Autodesk Inventor part; units mm, degrees
ref_plane "XZ Plane" through (0, 0, 0) normal (0, 1, 0) x (-1, 0, 0)
ref_plane "XY Plane" through (0, 0, 0) normal (0, 0, 1) x (1, 0, 0)
sketch "Sketch1" plane through (0, 0, 0) normal (0, 0, 1) x (1, 0, 0)
  circle A0 centre (0, 0) radius 7.9375
  dimension "d0" = 15.875
extrude "Extrusion1" add sketch "Sketch1" along normal blind 58.039
sketch "Sketch2" plane through (0, 0, 0) normal (0, 0, -1) x (-1, 0, 0)
  circle A0 centre (0, 0) radius 82.55
  dimension "d3" = 165.1
extrude "Extrusion2" add sketch "Sketch2" along normal blind 45.4533
sketch "Sketch3" plane through (0, 0, -45.4533) normal (0, 0, -1) x (-1, 0, 0)
  circle A0 centre (0, 0) radius 67.2719
  circle A1 centre (0, 0) radius 53.975
  dimension "d6" = 134.5438
  dimension "d20" = 107.95
ref_plane "Work Plane3" through (0, 0, -45.4533) normal (0, 0, -1) x (-1, 0, 0)
sketch "Sketch4" plane through (0, 0, -45.4533) normal (0, 0, -1) x (-1, 0, 0)
  point P0 (0, 0)
ref_plane "Work Plane1" through (7.9375, 0, 0) normal (1, 0, 0) x (0, 1, 0)
sketch "Sketch5" plane through (7.9375, 0, 0) normal (1, 0, 0) x (0, 1, 0)
  line L0 (-7.9375, 0) -> (-7.9375, 58.039)
  line L1 (7.9375, 58.039) -> (-7.9375, 58.039)
  line L2 (7.9375, 58.039) -> (-7.9375, 58.039)
  line L3 (7.9375, 0) -> (-7.9375, 0)
  line L4 (7.9375, 0) -> (7.9375, 58.039)
  line L5 (5.8928, 55.245) -> (5.8928, 10.8077)
  line L6 (5.8928, 55.245) -> (7.9375, 55.245)
  line L7 (5.8928, 10.8077) -> (7.9375, 10.8077)
  point P0 (0, 0)
  dimension "d9" = 13.8303
  dimension "d10" = 2.794
  dimension "d11" = 10.8077
extrude "Extrusion4" cut sketch "Sketch5" against normal blind 50.8 contours L7 L5 L6 L4
sketch "Sketch6" plane through (0, 0, 58.039) normal (0, 0, 1) x (1, 0, 0)
  circle A0 centre (0, 0) radius 3.2512
  dimension "d14" = 6.5024
ref_plane "Work Plane2" through (0, 0, -49.2633) normal (-1, 0, 0) x (0, 0, 1)
extrude "Extrusion6" add sketch "Sketch3" along normal blind 10.16 draft -25
extrude "Extrusion7" add sketch "Sketch3" along normal blind 10.16 draft 25 contours A1
sketch "Sketch8" plane through (0, 0, -49.2633) normal (-1, 0, 0) x (0, 0, 1)
  line L0 (49.2633, 82.55) -> (3.81, 82.55)
  line L1 (26.5367, 82.55) -> (26.5367, 46.429)
  arc A0 (49.2633, 69.85) -> (26.5367, 82.55) centre (26.5367, 55.8653) ccw
  line L2 (49.2633, 82.55) -> (49.2633, -82.55)
  arc A1 (26.5367, 82.55) -> (3.81, 69.85) centre (26.5367, 55.8653) ccw
  line L3 (49.2633, 82.55) -> (3.81, 82.55)
  line L4 (3.81, 82.55) -> (3.81, -82.55)
  line L5 (-29.0805, 0) -> (130.0328, 0)
  point P0 (49.2633, 0)
  dimension "d25" = 0
  dimension "d26" = 12.7
revolve "Revolution2" cut sketch "Sketch8" angle 360 about axis through (0, 0, -49.2633) along (0, 0, 1) contours L2 A0 L0 | A1 L4 L0
extrude "Extrusion8" cut sketch "Sketch6" against normal blind 50.8
properties part number "Wheel"
The listing builds one solid part. Answer for the finished solid, in the listing's coordinates (mm). A direction names the side the tool comes from. Coordinates: 2 decimals unless noted, no trailing zeros. Write each loop counter-clockwise with the first axis right and the second up, starting at its lowest first coordinate (ties: lowest second). Pieces come first, ordered by that corner, then holes.
Q1. Section A-A, the plane y = 0 is taken. Write down the section's boundary in (x, z).
Returned:
outline: (-82.55, -22.73) arc R26.68 ccw to (-69.85, -45.45) - (-67.27, -45.45) - (-62.53, -55.61) - (62.53, -55.61) - (67.27, -45.45) - (69.85, -45.45) arc R26.68 ccw to (82.55, -22.73) arc R26.68 ccw to (69.85, 0) - (7.94, 0) - (7.94, 58.04) - (3.25, 58.04) - (3.25, 7.24) - (-3.25, 7.24) - (-3.25, 58.04) - (-7.94, 58.04) - (-7.94, 0) - (-69.85, 0) arc R26.68 ccw to start
Q2. Section C-C, the plane z = 46 is taken. Write down the section's boundary in (x, y) (1 decimal).
Returned:
outline: (-5.3, 5.9) arc R7.9 ccw (long way) to (5.3, 5.9) - close; hole circle Ø6.5 at (0, 0)
Q3. Given P1, Ø10, axis at x = -16.5, y = -35.5, coming from the +Z side; P2, Ø3, axis at y = 19, z = -17, coming from the -X side; P3, Ø1, axis at x = 61, z = -13, coming from the +Y side, each flat-ended and moving along its own axis, determine where each tip first touches the part or whether it passes through.
Returned:
P1: stops at z = 0
P2: stops at x = -80.16
P3: stops at y = 53.5
Q4. The mould has two halves that part along Y. Classify faces 4 (the flat face through (-15, 1, 0)), 5 (the cylindrical face through (-0.423, 3.224, 32.995)), 6 (the cylindrical face through (-1.03, -7.87, 28.61)): released by +Y, released by -Y, zero draft, split by the parting line, or undercut.
Returned:
face 4: zero draft
face 5: undercut
face 6: split by the parting line
Q5. Section D-D, the plane z = -41 is taken. Write down the section's boundary in (x, y), then the cut area to 3 significant figures.
Returned:
outline: circle Ø150.62 at (0, 0)
area: 17,800 mm2
Q6. Find the intervals of material crossed by line 1 along Y through (x, z) = (0, 38); line 2 along Z through (x, y) = (21.5, -12); line 3 along Y through (x, z) = (15.5, -27.5), in increasing order.
Returned:
line 1: y = -7.94 to -3.25, 3.25 to 5.89
line 2: z = -55.61 to 0
line 3: y = -80.64 to 80.64
Q7. Which of the six approach directions +Z, -Z, +X, -X, +Y, -Y give full straight-line access (tool end or side, diameter ignored) to faces 1 (the flat face through (0, 0, 7.239)), 2 (the flat face through (37, 57, -45.453)), 3 (the flat face through (0, 5.893, 33))?
Returned:
face 1: +Z
face 2: -Z
face 3: +X, -X, +Y
